Verification items for the finished model (mm, model axes). Round coordinates to 2 decimals unless told otherwise and drop trailing zeros. Order: outer loops, then holes, each group sorted by start corner. A loop starts at its lowest first (then second) coordinate and runs counter-clockwise, first axis right, second up. Notation, with made-up numbers: M 72.5,50.5 L 87.5,50.5 A25 ccw 87.5,82.5 Z; hole C -16,-19 d1. An arc over 180 degrees is marked long. Write item = value, one per line. Start each with the question number.
from build123d import *

# Parameters (mm, degrees)
SKETCH1_W                       = 230
SKETCH1_H                       = 50
BOSS_EXTRUDE1_DEPTH             = 10
M10_CLEARANCE_HOLE1_D           = 11
M10_CLEARANCE_HOLE1_CSINK_D     = 11.05
M10_CLEARANCE_HOLE1_CSINK_ANGLE = 90


with BuildPart() as part:
    # Sketch1 → Boss-Extrude1 (new body)
    with BuildSketch(Plane(origin=(0, 0, 0), x_dir=(1, 0, 0), z_dir=(0, 1, 0))):
        Rectangle(SKETCH1_W, SKETCH1_H)
    extrude(amount=BOSS_EXTRUDE1_DEPTH)

    # M10 Clearance Hole1 (through all)
    with Locations(Plane(origin=(0, 10, 0), x_dir=(1, 0, 0), z_dir=(0, 1, 0))):
        with Locations((-90, 0)):
            CounterSinkHole(M10_CLEARANCE_HOLE1_D / 2, M10_CLEARANCE_HOLE1_CSINK_D / 2, counter_sink_angle=M10_CLEARANCE_HOLE1_CSINK_ANGLE)


solid = part.part
1) Cross-section at A-A, the plane x = -90. Enter the section's corners in (y, z) (3 decimals), then the cut area to 3 significant figures.
2) Cross-section at B-B, the plane z = 0. Enter the section's corners in (x, y) (3 decimals), then the cut area to 3 significant figures.
3) Scan lines: probe 1 along Z at (x, y) = (-90, 7); probe 2 along X at (y, z) = (5.75, -0.5); probe 3 along X at (y, z) = (5.5, 3.5). Record each from-to range of solid material in increasing order.
4) Release check for a two-part mould opening along Z. For faces 1 (the flat face through (-2, 5, 25)), 2 (the flat face through (115, 5, 0)), 3 (the flat face through (-2, 5, -25)), 4 (the cylindrical face through (-84.505, 4.918, -0.242)) record: pulls with the +Z half, pulls with the -Z half, needs draft (parallel to the pull), parting line crosses it, or undercut.
Geometry results:
q1.outline = M 0,-25 L 10,-25 L 10,-5.525 L 9.975,-5.5 L 0,-5.5 Z; M 0,5.5 L 9.975,5.5 L 10,5.525 L 10,25 L 0,25 Z
q1.area = 390 mm^2
q2.outline = M -115,0 L -95.5,0 L -95.5,9.975 L -95.525,10 L -115,10 Z; M -84.5,0 L 115,0 L 115,10 L -84.475,10 L -84.5,9.975 Z
q2.area = 2,190 mm^2
q3.probe_1 = -25 to -5.5, 5.5 to 25
q3.probe_2 = -115 to -95.48, -84.52 to 115
q3.probe_3 = -115 to -94.24, -85.76 to 115
q4.face_1 = pulls with the +Z half
q4.face_2 = needs draft
q4.face_3 = pulls with the -Z half
q4.face_4 = undercut
